from build123d import *

# Parameters (mm, degrees)
F0_W     = 6
F0_H     = 10
F1_DEPTH = 3


with BuildPart() as f1:
    # F0 (on Top) → F1 (new body)
    with BuildSketch(Plane.XY):
        Polygon((48.401362, -61.559224), (75.341128, 21.352851), (73.503144, 27.009584), (2.973921, 78.252065), (-2.973921, 78.252065), (-73.503144, 27.009584), (-75.341128, 21.352851), (-48.401362, -61.559224), (-43.589457, -65.055277), (43.589457, -65.055277), align=None)
        Polygon((-45.365977, -57.337006), (-39.488125, -49.246836), (-34.634023, -52.773548), (-40.511875, -60.863718), align=None, mode=Mode.SUBTRACT)
        Polygon((40.511875, -60.863718), (34.634023, -52.773548), (39.488125, -49.246836), (45.365977, -57.337006), align=None, mode=Mode.SUBTRACT)
        Polygon((-68.549591, 25.427499), (-59.039026, 22.337329), (-60.893128, 16.63099), (-70.403693, 19.72116), align=None, mode=Mode.SUBTRACT)
        Polygon((70.403693, 19.72116), (60.893128, 16.63099), (59.039026, 22.337329), (68.549591, 25.427499), align=None, mode=Mode.SUBTRACT)
        with Locations((0, 68.052065)):
            Rectangle(F0_W, F0_H, mode=Mode.SUBTRACT)
    extrude(amount=F1_DEPTH)


solid = f1.part
Design review of the part built by this model. Coordinates are the model's own, in mm. A direction names the side the tool comes from. Give positions to 0.01 mm unless a question says otherwise; leave off trailing zeros. Write each loop counter-clockwise with the first axis right and the second up, starting at its lowest first coordinate (ties: lowest second). Pieces come first, ordered by that corner, then holes. Notation, with made-up numbers: M 19.25,6.25 L 41.25,6.25 A30 ccw 41.25,38.25 Z; hole C 8,-29 d3. An arc over 180 degrees is marked long. Answer as a JSON object with one key per item and string values. Group by question number.
1) We need section D-D (y = -21). Give the boundary of the cut face in (x, z).
2) Tool access review of faces 4 (the face through (61.683, -20.684, 1.479)), 5 (the face through (42.97, -59.08, 1.48)): name each direction out of +Z, -Z, +X, -X, +Y, -Y from which nothing blocks a thin tool from reaching the whole face with its end or side.
3) We need section B-B (z = 1.85). Count the separate pieces of the cut face and the enclosed holes in it, and give its area (3 significant figures).
4) We need section A-A (x = 36.5). Give the boundary of the cut face in (y, z).
5) Clearance check with flat-ended pins moving along their axes: pin 1 Ø1.5 at (y, z) = (70, 1) entering from -X; pin 2 Ø2 at (x, y) = (-36, 4.5) entering from -Z; pin 3 Ø1.5 at (y, z) = (68, 1.5) entering from +X. State where each tip first meets the part, or that it passes through.
6) For line 1 along X through (y, z) = (21, 1.4); line 2 along X through (y, z) = (21.5, 1.3); line 3 along Y through (x, z) = (-42, 1.55), list the stretches that pass through material, from the lowest coordinate up.
7) Mouldability with a two-part tool opening along X and no side actions: class faces 1 (the face through (-62.06, -19.52, 1.48)), 2 (the face through (-1, -8, 0)), 3 (the face through (42.39, -53.24, 1.48)) as released by +X, released by -X, zero draft, split by the parting line, or undercut.
8) We need section C-C (y = 68). Give the boundary of the cut face in (x, z).
Answer key:
{
 "1": {"outline": "M -61.58,0 L 61.58,0 L 61.58,3 L -61.58,3 Z"},
 "2": {"face 4": "+Z, -Z, +X, -Y", "face 5": "+Z, -Z"},
 "3": {"separate pieces": "1", "enclosed holes": "5", "area": "15,000 mm²"},
 "4": {"outline": "M -65.06,0 L -55.34,0 L -55.34,3 L -65.06,3 Z; M -51.42,0 L 53.89,0 L 53.89,3 L -51.42,3 Z"},
 "5": {"pin 1": "stops at x = -15.36", "pin 2": "stops at z = 0", "pin 3": "stops at x = 18.12"},
 "6": {"line 1": "x = -75.23 to -69.99, -59.47 to 59.47, 69.99 to 75.23", "line 2": "x = -75.29 to -69.83, -59.31 to 59.31, 69.83 to 75.29", "line 3": "y = -65.06 to -59.78, -52.7 to 49.9"},
 "7": {"face 1": "released by -X", "face 2": "zero draft", "face 3": "undercut"},
 "8": {"outline": "M -17.08,0 L -3,0 L -3,3 L -17.08,3 Z; M 3,0 L 17.08,0 L 17.08,3 L 3,3 Z"}
}
